Verification items for the finished model (mm, model axes). Round coordinates to 2 decimals unless told otherwise and drop trailing zeros. Loops run counter-clockwise (first coordinate to the right, second up) from the corner with the lowest first, then second, coordinate; pieces in that order, holes last. Notation, with made-up numbers: (62, 18.5) - (76, 18.5) arc R14 cw to (76, 27.5) - close; hole circle Ø8 at (58, -13). An arc over 180 degrees is marked (long way). Use CSV: the item, a comma, the result in double quotes.
Autodesk Inventor part; units mm, degrees
ref_plane "YZ Plane" through (0, 0, 0) normal (1, 0, 0) x (0, 1, 0)
ref_plane "XZ Plane" through (0, 0, 0) normal (0, 1, 0) x (-1, 0, 0)
ref_plane "XY Plane" through (0, 0, 0) normal (0, 0, 1) x (1, 0, 0)
sketch "Sketch12" plane through (0, 0, 0) normal (0, 0, 1) x (1, 0, 0)
  line L0 (-20, 26) -> (20, 26)
  line L1 (20, 26) -> (20, 0)
  line L2 (20, 0) -> (-20, 0)
  line L3 (-20, 0) -> (-20, 26)
  circle A0 centre (0, 15) radius 5.5
  point P0 (0, 0)
  point P1 (0, 0)
  dimension "d73" = 40
  dimension "d74" = 11
  dimension "d77" = 15
  dimension "d78" = 26
extrude "Plate3" add sketch "Sketch12" along normal blind 3
fillet "Corner Round1" radius 6 2 edges at (-20, 26, 1.5) (20, 26, 1.5)
equation "\"d75\" = Thickness"
equation "\"BendRadius\" = Thickness"
equation "\"BendReliefWidth\" = Thickness"
equation "\"BendReliefDepth\" = 0.5 * Thickness"
equation "\"CornerReliefSize\" = 4 * Thickness"
equation "\"MinimumRemnant\" = 2 * Thickness"
equation "\"TransitionRadius\" = BendRadius"
equation "\"JacobiRadiusSize\" = BendRadius"
equation "\"GapSize\" = Thickness"
properties part number "ДМФ 094 Постель НОС крепление v2.0"
1) Cross-section at D-D, the plane y = 22.5. Record the cut outline in (x, z).
Returned:
outline,"(-19.45, 0) - (19.45, 0) - (19.45, 3) - (-19.45, 3) - close"
2) Cross-section at A-A, the plane y = 15. Record the cut outline in (x, z), then the cut area to 3 significant figures.
Returned:
outline,"(-20, 0) - (-5.5, 0) - (-5.5, 3) - (-20, 3) - close; (5.5, 0) - (20, 0) - (20, 3) - (5.5, 3) - close"
area,"87.0 mm²"
3) Thickness scan on probe 1 along Y at (x, z) = (0, 0.8); probe 2 along X at (y, z) = (11.25, 1.55); probe 3 along Y at (x, z) = (-2, 1.25). Record the ranges inside material, lowest first. Write a range as [from, to].
Returned:
probe 1,"y = [0, 9.5], [20.5, 26]"
probe 2,"x = [-20, -4.02], [4.02, 20]"
probe 3,"y = [0, 9.88], [20.12, 26]"
4) Cross-section at B-B, the plane x = 0. Record the cut outline in (y, z).
Returned:
outline,"(0, 0) - (9.5, 0) - (9.5, 3) - (0, 3) - close; (20.5, 0) - (26, 0) - (26, 3) - (20.5, 3) - close"
5) Cross-section at C-C, the plane z = 2.2. Record the cut outline in (x, y).
Returned:
outline,"(-20, 0) - (20, 0) - (20, 20) arc R6 ccw to (14, 26) - (-14, 26) arc R6 ccw to (-20, 20) - close; hole circle Ø11 at (0, 15)"
6) Mould release check, pull along Y, two halves, no side actions. Record for faces 1 (the face through (18.289, 24.196, 1.521)), 2 (the face through (-1.19, 20.37, 1.48)), 3 (the face through (-20, 10, 1)): +Y half, -Y half, draft (parallel to the pull), parting line (faces both ways), or undercut.
Returned:
face 1,"+Y half"
face 2,"undercut"
face 3,"draft"
